The drawing under review shows one solid part. Ordinate dimensions are in mm from its lowest x, y, z. Coordinates: 2 decimals unless noted, no trailing zeros. Order: outer loops, then holes, each group sorted by start corner. A loop starts at its lowest first (then second) coordinate and runs counter-clockwise, first axis right, second up.
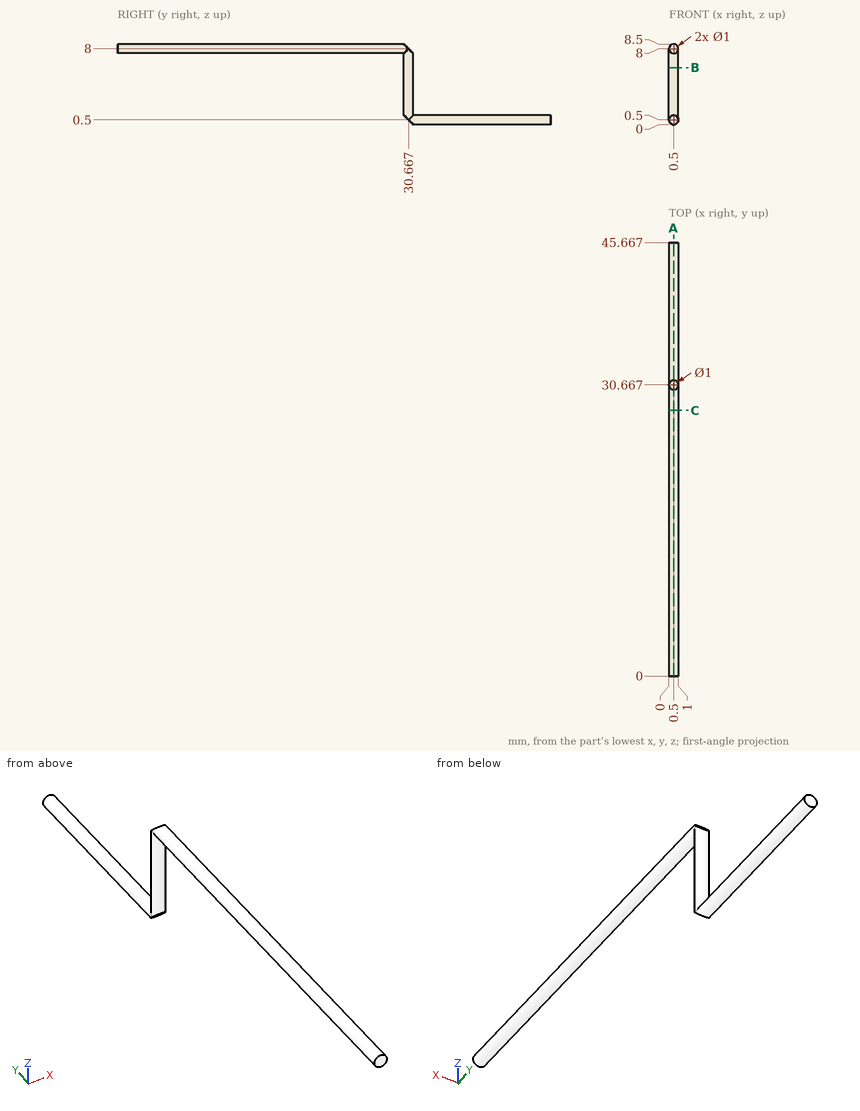
(1) We need section C-C, the plane y = 28. Write out the cut boundary in (x, z).
A:
outline: circle Ø1 at (0.5, 8)
(2) We need section A-A, the plane x = 0.5. Write out the cut boundary in (y, z).
A:
outline: (0, 7.5) - (30.17, 7.5) - (30.17, 1) - (31.17, 0) - (45.67, 0) - (45.67, 1) - (31.17, 1) - (31.17, 7.5) - (30.17, 8.5) - (0, 8.5) - close
(3) Wall thickness on probe 1 along Z at (x, y) = (0.45, 34); probe 2 along Y at (x, z) = (0.55, 4.5); probe 3 along Z at (x, y) = (0.45, 11.5): over which ranges is each line inside the solid? List them lowest first.
A:
probe 1: z = 0 to 1
probe 2: y = 30.17 to 31.16
probe 3: z = 7.5 to 8.5
(4) We need section B-B, the plane z = 6. Write out the cut boundary in (x, y).
A:
outline: circle Ø1 at (0.5, 30.67)
